Answer from the drawing. Dimensions are ordinates in mm from the lowest x, y and z of the part. Coordinates: 2 decimals unless noted, no trailing zeros. Write each loop counter-clockwise with the first axis right and the second up, starting at its lowest first coordinate (ties: lowest second). Pieces come first, ordered by that corner, then holes.
(1) Section D-D on y = 145 is taken. Write down the section's boundary in (x, z), then the cut area to 3 significant figures.
(2) Find the intervals of material crossed by probe 1 along Z at (x, y) = (9.75, 99); probe 2 along Y at (x, z) = (4.75, 0.75); probe 3 along Y at (x, z) = (4.5, 1.75), in increasing order.
(3) Section B-B on y = 120 is taken. Write down the section's boundary in (x, z).
(4) Section A-A on x = 5 is taken. State how many separate pieces and enclosed holes the cut face has, then the cut area to 3 significant figures.
(5) Section C-C on z = 5.1 is taken. Write down the section's boundary in (x, y), then the cut area to 3 significant figures.
(6) Given pin 1 (6 mm diameter, centred on x = 5, y = 60, fed in from -Z); pin 2 (1 mm diameter, centred on x = 5.5, z = 1.5, fed in from +Y), each flat-ended and moving along its own axis, determine where each tip first touches the part or whether it passes through.
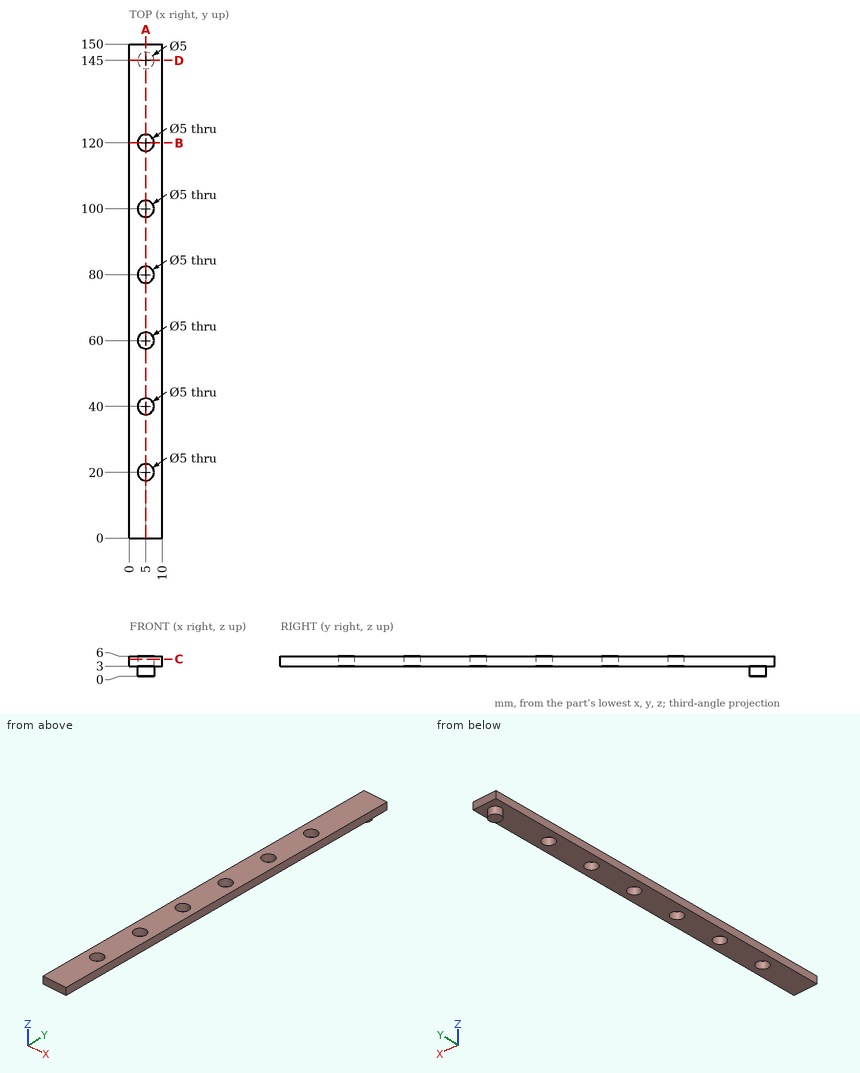
Response:
1. outline: (0, 3) - (2.5, 3) - (2.5, 0) - (7.5, 0) - (7.5, 3) - (10, 3) - (10, 6) - (0, 6) - close
1. area: 45.0 mm2
2. probe 1: z = 3 to 6
2. probe 2: y = 142.51 to 147.49
2. probe 3: y = 142.55 to 147.45
3. outline: (0, 3) - (2.5, 3) - (2.5, 6) - (0, 6) - close; (7.5, 3) - (10, 3) - (10, 6) - (7.5, 6) - close
4. separate pieces: 7
4. enclosed holes: 0
4. area: 375 mm2
5. outline: (0, 0) - (10, 0) - (10, 150) - (0, 150) - close; hole circle Ø5 at (5, 20); hole circle Ø5 at (5, 40); hole circle Ø5 at (5, 60); hole circle Ø5 at (5, 80); hole circle Ø5 at (5, 100); hole circle Ø5 at (5, 120)
5. area: 1,380 mm2
6. pin 1: stops at z = 3
6. pin 2: stops at y = 147.5
